```python
from build123d import *

# Parameters (mm, degrees)
BASE_EXTRUDE_DEPTH = 12.7


with BuildPart() as part:
    # Sketch1 → Base-Extrude (new, symmetric)
    with BuildSketch(Plane.XY):
        with BuildLine():
            Line((-41.275, 39.7764), (-41.275, 34.34565134))
            ThreePointArc((-41.275, 34.34565134), (-39.7764, 31.75), (-41.275, 29.15434866))
            Line((-41.275, 29.15434866), (-41.275, 12.12065134))
            ThreePointArc((-41.275, 12.12065134), (-39.7764, 9.525), (-41.275, 6.92934866))
            Line((-41.275, 6.92934866), (-41.275, 1.4986))
            ThreePointArc((-41.275, 1.4986), (-40.836070222, 0.438929778), (-39.7764, 0))
            Line((-39.7764, 0), (-1.4986, 0))
            ThreePointArc((-1.4986, 0), (-0.438929778, 0.438929778), (0, 1.4986))
            Line((0, 1.4986), (0, 6.92934866))
            ThreePointArc((0, 6.92934866), (-1.4986, 9.525), (0, 12.12065134))
            Line((0, 12.12065134), (0, 29.15434866))
            ThreePointArc((0, 29.15434866), (-1.4986, 31.75), (0, 34.34565134))
            Line((0, 34.34565134), (0, 39.7764))
            ThreePointArc((0, 39.7764), (-0.438929778, 40.836070222), (-1.4986, 41.275))
            Line((-1.4986, 41.275), (-8.0264, 41.275))
            ThreePointArc((-8.0264, 41.275), (-9.086070222, 40.836070222), (-9.525, 39.7764))
            Line((-9.525, 39.7764), (-9.525, 34.925))
            Line((-9.525, 34.925), (-8.0264, 34.925))
            Line((-8.0264, 34.925), (-8.0264, 39.7764))
            Line((-8.0264, 39.7764), (-1.4986, 39.7764))
            Line((-1.4986, 39.7764), (-1.4986, 35.100971471))
            ThreePointArc((-1.4986, 35.100971471), (-2.9972, 31.75), (-1.4986, 28.399028529))
            Line((-1.4986, 28.399028529), (-1.4986, 12.875971471))
            ThreePointArc((-1.4986, 12.875971471), (-2.9972, 9.525), (-1.4986, 6.174028529))
            Line((-1.4986, 6.174028529), (-1.4986, 1.4986))
            Line((-1.4986, 1.4986), (-39.7764, 1.4986))
            Line((-39.7764, 1.4986), (-39.7764, 6.174028529))
            ThreePointArc((-39.7764, 6.174028529), (-38.2778, 9.525), (-39.7764, 12.875971471))
            Line((-39.7764, 12.875971471), (-39.7764, 28.399028529))
            ThreePointArc((-39.7764, 28.399028529), (-38.2778, 31.75), (-39.7764, 35.100971471))
            Line((-39.7764, 35.100971471), (-39.7764, 39.7764))
            Line((-39.7764, 39.7764), (-33.2486, 39.7764))
            Line((-33.2486, 39.7764), (-33.2486, 34.925))
            Line((-33.2486, 34.925), (-31.75, 34.925))
            Line((-31.75, 34.925), (-31.75, 39.7764))
            ThreePointArc((-31.75, 39.7764), (-32.188929778, 40.836070222), (-33.2486, 41.275))
            Line((-33.2486, 41.275), (-39.7764, 41.275))
            ThreePointArc((-39.7764, 41.275), (-40.836070222, 40.836070222), (-41.275, 39.7764))
        make_face()
    base_extrude = extrude(amount=BASE_EXTRUDE_DEPTH, both=True)

    # Mirror1: Base-Extrude across plane
    add(base_extrude.mirror(Plane.ZX))


solid = part.part
```
Can you work these out from the model? Positions are in its coordinate system, mm. A direction names the side the tool comes from. Round coordinates to 2 decimals unless told otherwise and drop trailing zeros. Loops run counter-clockwise (first coordinate to the right, second up) from the corner with the lowest first, then second, coordinate; pieces in that order, holes last. Notation, with made-up numbers: M 85,44.25 L 92,44.25 A21 ccw 92,65.25 Z; hole C 49,65.25 d9. An arc over 180 degrees is marked long. Answer as a JSON object with one key per item and string values. Group by question number.
Q1. Imagine slicing it at C-C, the plane y = -9. Please give me the cut outline in (x, z).
Q2. Imagine slicing it at B-B, the plane y = 26. Please give me the cut outline in (x, z) (3 decimals), then the cut area to 3 significant figures.
Q3. We'd pull the mould along Y, two halves only. Please class faces 1 (the flat face through (-9.525, -37, 0)), 2 (the flat face through (-39.776, 37, 0)): +Y half, -Y half, draft (parallel to the pull), parting line (faces both ways), or undercut.
Q4. On a 3-axis mill with a long thin cutter (end or side, diameter ignored), from which of +Z, -Z, +X, -X, +Y, -Y can I reach the whole of each face in a straight line? I mean faces 3 (the cylindrical face through (-39.777, -31.794, 0.178)), 4 (the flat face through (-5, -39.776, 0)), 5 (the flat face through (-31.75, 37, 0)). Say none if no direction works.
Q5. Imagine slicing it at D-D, the plane x = -23.5. Please give me the cut outline in (y, z), then the cut area to 3 significant figures.
Q6. Please list where these lines run through material, in increasing order: L1, parallel to Y at x = -33.5, z = -4 (3 decimals); L2, parallel to X at y = -36, z = 2.25 (3 decimals); L3, parallel to X at y = -22.5, z = -1.25 (3 decimals).
Q7. Will these pins go through, and if not, where does the flat tip stop? pin 1 (1 mm diameter, centred on x = -15, z = 2, fed in from +Y); pin 2 (0.7 mm diameter, centred on x = -32.5, z = -5, fed in from -Y); pin 3 (10 mm diameter, centred on y = 12, z = -4, fed in from -X) (3 decimals); pin 4 (0.7 mm diameter, centred on x = -8.5, z = -5, fed in from +Y).
Q8. Imagine slicing it at A-A, the plane x = -36.5. Please give me the cut outline in (y, z) (3 decimals), then the cut area to 3 significant figures.
Findings:
{
 "1": {"outline": "M -39.82,-12.7 L -38.31,-12.7 L -38.31,12.7 L -39.82,12.7 Z; M -2.97,-12.7 L -1.45,-12.7 L -1.45,12.7 L -2.97,12.7 Z"},
 "2": {"outline": "M -41.275,-12.7 L -39.776,-12.7 L -39.776,12.7 L -41.275,12.7 Z; M -1.499,-12.7 L 0,-12.7 L 0,12.7 L -1.499,12.7 Z", "area": "76.1 mm2"},
 "3": {"face 1": "draft", "face 2": "undercut"},
 "4": {"face 3": "+Z, -Z, -X", "face 4": "+Z, -Z", "face 5": "+Z, -Z, +Y"},
 "5": {"outline": "M -1.5,-12.7 L 1.5,-12.7 L 1.5,12.7 L -1.5,12.7 Z", "area": "76.1 mm2"},
 "6": {"L1": "y = -41.275 to -39.776, -1.499 to 1.499, 39.776 to 41.275", "L2": "x = -41.275 to -39.776, -33.249 to -31.75, -9.525 to -8.026, -1.499 to 0", "L3": "x = -41.275 to -39.776, -1.499 to 0"},
 "7": {"pin 1": "stops at y = 1.5", "pin 2": "stops at y = -41.22", "pin 3": "stops at x = -41.275", "pin 4": "stops at y = 41.27"},
 "8": {"outline": "M -41.275,-12.7 L -39.776,-12.7 L -39.776,12.7 L -41.275,12.7 Z; M -1.499,-12.7 L 1.499,-12.7 L 1.499,12.7 L -1.499,12.7 Z; M 39.776,-12.7 L 41.275,-12.7 L 41.275,12.7 L 39.776,12.7 Z", "area": "152 mm2"}
}
